Source: CAD feature listing. Evaluate the final solid. Frame: model axes, mm. Give positions to 0.01 mm unless a question says otherwise; leave off trailing zeros. Order: outer loops, then holes, each group sorted by start corner. A loop starts at its lowest first (then second) coordinate and runs counter-clockwise, first axis right, second up. Notation, with made-up numbers: (59, 52) -> (117, 52) arc R9 cw to (117, 56) -> close; hole circle Ø10 at (-6.75, 28.25). An arc over 180 degrees is marked (long way). Use CSV: the item, a comma, the result in double quotes.
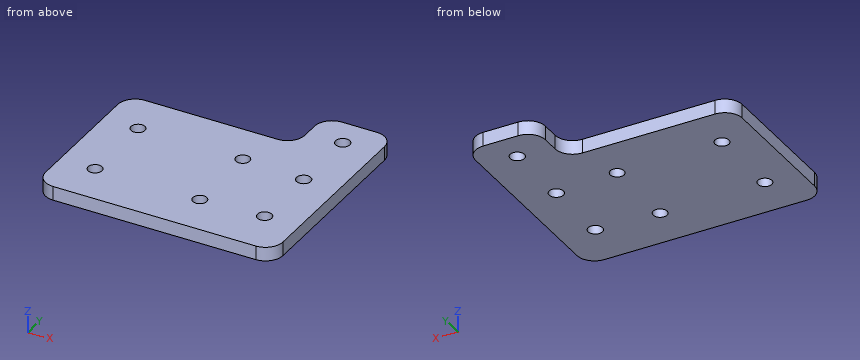
```python
from build123d import *

# Parameters (mm, degrees)
SKETCH_1_W          = 68
SKETCH_1_H          = 47
EXTRUDE_1_DEPTH     = 4
SKETCH_2_R          = 2
SKETCH_2_R_2        = 2.05
CUT_EXTRUDE_1_DEPTH = 4
SKETCH_5_W          = 20
SKETCH_5_H          = 15
EXTRUDE_3_DEPTH     = 4
SKETCH_6_R          = 2.05
CUT_EXTRUDE_3_DEPTH = 12
FILLET_3_R          = 5


with BuildPart() as part:
    # 草图1 → 凸台-拉伸1 (new body)
    with BuildSketch(Plane.XY):
        with Locations((34, 23.5)):
            Rectangle(SKETCH_1_W, SKETCH_1_H)
    extrude(amount=EXTRUDE_1_DEPTH)

    # 草图2 → 切除-拉伸1 (cut)
    with BuildSketch(Plane.XY.offset(4)):
        with Locations((10, 34.5)):
            Circle(SKETCH_2_R)
        with Locations(Location((10, 12.5, 0), (0, 0, 180))):
            Circle(SKETCH_2_R)
        with Locations((40, 34.5)):
            Circle(SKETCH_2_R)
        with Locations(Location((40, 12.5, 0), (0, 0, 180))):
            Circle(SKETCH_2_R)
        with Locations((58, 33.5)):
            Circle(SKETCH_2_R_2)
        with Locations(Location((58, 13.5, 0), (0, 0, 180))):
            Circle(SKETCH_2_R_2)
    extrude(amount=-CUT_EXTRUDE_1_DEPTH, mode=Mode.SUBTRACT)

    # 草图5 → 凸台-拉伸3 (add)
    with BuildSketch(Plane.XY.offset(4)):
        with Locations((58, 54.5)):
            Rectangle(SKETCH_5_W, SKETCH_5_H)
    extrude(amount=-EXTRUDE_3_DEPTH)

    # 草图6 → 切除-拉伸3 (cut)
    with BuildSketch(Plane.XY.offset(4)):
        with Locations((58, 33.5)):
            Circle(SKETCH_6_R)
        with Locations((58, 53.5)):
            Circle(SKETCH_6_R)
    extrude(amount=-CUT_EXTRUDE_3_DEPTH, mode=Mode.SUBTRACT)

    # 圆角3
    fillet_3_edges = [part.edges().sort_by_distance(p)[0] for p in [
        (68, 62, 2),
        (48, 47, 2),
        (48, 62, 2),
        (0, 47, 2),
        (68, 0, 2),
        (0, 0, 2),
    ]]
    fillet(fillet_3_edges, radius=FILLET_3_R)


solid = part.part
```
1. Section query B-B on x = 10. Return loops of the section in (y, z), plus the area to 3 significant figures.
Answer below:
outline,"(0, 0) -> (10.5, 0) -> (10.5, 4) -> (0, 4) -> close; (14.5, 0) -> (32.5, 0) -> (32.5, 4) -> (14.5, 4) -> close; (36.5, 0) -> (47, 0) -> (47, 4) -> (36.5, 4) -> close"
area,"156 mm²"
2. Ray query, line 1 along Y through (x, z) = (58, 2); line 2 along Y through (x, z) = (40, 2.55); line 3 along X through (y, z) = (12.5, 2.25). Return the intervals inside material, ascending.
Answer below:
line 1,"y = 0 to 11.45, 15.55 to 31.45, 35.55 to 51.45, 55.55 to 62"
line 2,"y = 0 to 10.5, 14.5 to 32.5, 36.5 to 47"
line 3,"x = 0 to 8, 12 to 38, 42 to 56.21, 59.79 to 68"
3. Section query D-D on z = 2.4. Return loops of the section in (x, y), plus the area to 3 significant figures.
Answer below:
outline,"(0, 5) arc R5 ccw to (5, 0) -> (63, 0) arc R5 ccw to (68, 5) -> (68, 57) arc R5 ccw to (63, 62) -> (53, 62) arc R5 ccw to (48, 57) -> (48, 52) arc R5 cw to (43, 47) -> (5, 47) arc R5 ccw to (0, 42) -> close; hole circle Ø4 at (10, 12.5); hole circle Ø4 at (10, 34.5); hole circle Ø4 at (40, 12.5); hole circle Ø4 at (40, 34.5); hole circle Ø4.1 at (58, 13.5); hole circle Ø4.1 at (58, 33.5); hole circle Ø4.1 at (58, 53.5)"
area,"3,380 mm²"
4. Section query A-A on y = 53.5. Return loops of the section in (x, z), plus the area to 3 significant figures.
Answer below:
outline,"(48, 0) -> (55.95, 0) -> (55.95, 4) -> (48, 4) -> close; (60.05, 0) -> (68, 0) -> (68, 4) -> (60.05, 4) -> close"
area,"63.6 mm²"
5. Pin query (flat end, axial travel): P1, Ø1.5, axis at x = 25.5, z = 0.5, coming from the +Y side; P2, Ø6.5, axis at x = 40, y = 12.5, coming from the -Z side. Return the tip coordinate at first contact, or that it passes through.
Answer below:
P1,"stops at y = 47"
P2,"stops at z = 0"
6. Section query C-C on x = 58. Return loops of the section in (y, z), plus the area to 3 significant figures.
Answer below:
outline,"(0, 0) -> (11.45, 0) -> (11.45, 4) -> (0, 4) -> close; (15.55, 0) -> (31.45, 0) -> (31.45, 4) -> (15.55, 4) -> close; (35.55, 0) -> (51.45, 0) -> (51.45, 4) -> (35.55, 4) -> close; (55.55, 0) -> (62, 0) -> (62, 4) -> (55.55, 4) -> close"
area,"199 mm²"
